For this review, take the finished solid that the model builds, in its own axes (mm). A direction names the side the tool comes from. Round coordinates to 2 decimals unless told otherwise and drop trailing zeros. Order: outer loops, then holes, each group sorted by start corner. A loop starts at its lowest first (then second) coordinate and runs counter-clockwise, first axis right, second up. Notation, with made-up numbers: M 39.25,25.5 L 46.25,25.5 A19 ccw 46.25,29.5 Z; hole C 12,72.25 d2. An arc over 180 degrees is marked long. Put each result on its own line as item: value.
Autodesk Inventor part; units mm, degrees
ref_plane "YZ Plane" through (0, 0, 0) normal (1, 0, 0) x (0, 1, 0)
ref_plane "XZ Plane" through (0, 0, 0) normal (0, 1, 0) x (-1, 0, 0)
ref_plane "XY Plane" through (0, 0, 0) normal (0, 0, 1) x (1, 0, 0)
sketch "Sketch1" plane through (0, 0, 0) normal (0, 1, 0) x (-1, 0, 0)
  line L0 (0, 0) -> (34, 0)
  line L1 (34, 0) -> (34, -2)
  line L2 (34, -2) -> (0, -2)
  line L3 (0, -2) -> (0, 0)
  line L4 (37, -5) -> (37, 3)
  line L5 (37, 3) -> (-3, 3)
  line L6 (-3, 3) -> (-3, -5)
  line L7 (-3, -5) -> (37, -5)
  dimension "d0" = 34
  dimension "d1" = 2
  dimension "d2" = 3
extrude "Extrusion1" add sketch "Sketch1" along normal blind 48 contours L0 L1 L2 L3 | L7 L6 L5 L4
sketch "Sketch3" plane through (0, 0, 0) normal (0, -1, 0) x (1, 0, 0)
  line L0 (-37, 3) -> (3, 3)
  line L1 (-37, 3) -> (3, 3)
  line L2 (3, 3) -> (3, 18)
  line L3 (3, 18) -> (-37, 18)
  line L4 (-37, 18) -> (-37, 3)
  line L5 (3, -5) -> (-37, -5)
  line L6 (-37, -5) -> (3, -5)
  line L7 (3, -5) -> (3, -20)
  line L8 (3, -20) -> (-37, -20)
  line L9 (-37, -20) -> (-37, -5)
  circle A0 centre (-27, -12.5) radius 3
  circle A1 centre (-27, 13.5) radius 3
  circle A2 centre (-7, -12.5) radius 3
  circle A3 centre (-7, 13.5) radius 3
  point P0 (0, 0)
  point P1 (3, -5)
  dimension "d5" = 40
  dimension "d6" = 15
  dimension "d7" = 40
  dimension "d8" = 15
  dimension "d9" = 6
  dimension "d10" = 10
  dimension "d11" = 7.5
  dimension "d14" = 26
  dimension "d17" = 20
extrude "Extrusion2" add sketch "Sketch3" against normal blind 6 contours L4 L3 L2 L0
sketch "Sketch5" plane through (0, 48, 0) normal (0, 1, 0) x (1, 0, 0)
  line L0 (3, 5) -> (-37, 5)
  line L1 (-37, 5) -> (3, 5)
  line L2 (3, 5) -> (3, 17)
  line L3 (3, 17) -> (-37, 17)
  line L4 (-37, 17) -> (-37, 5)
  line L5 (-32, 13) -> (-22, 13) construction
  line L6 (-32, 11.41) -> (-22, 11.41)
  line L7 (-22, 14.59) -> (-32, 14.59)
  arc A0 (-32, 14.59) -> (-32, 11.41) centre (-32, 13) ccw
  arc A1 (-22, 11.41) -> (-22, 14.59) centre (-22, 13) ccw
  line L8 (-32, 13) -> (-22, 13) construction
  line L9 (-22, 13) -> (-10.76, 13)
  line L10 (-22, 13) -> (-10.76, 13) construction
  line L11 (-10.76, 13) -> (-0.76, 13) construction
  line L12 (-10.76, 11.41) -> (-0.76, 11.41)
  line L13 (-0.76, 14.59) -> (-10.76, 14.59)
  arc A2 (-10.76, 14.59) -> (-10.76, 11.41) centre (-10.76, 13) ccw
  arc A3 (-0.76, 11.41) -> (-0.76, 14.59) centre (-0.76, 13) ccw
  point P0 (0, 0)
  point P1 (-27, 13)
  point P2 (-5.76, 13)
  point P3 (3, 5)
  dimension "d40" = 40
  dimension "d41" = 12
  dimension "d43" = 10
  dimension "d44" = 0
  dimension "d45" = 3.18
  dimension "d46" = 11.24
  dimension "d47" = 0
  dimension "d48" = 10
  dimension "d49" = 3.18
  dimension "d57" = 4
  dimension "d58" = 10
extrude "Extrusion4" add sketch "Sketch5" against normal blind 6
fillet "Fillet1" radius 3 1 edges at (-17, 42, -5)
fillet "Fillet2" radius 3 2 edges at (-17, 48, 3) (-17, 6, 3)
fillet "Fillet3" radius 3 1 edges at (-17, 6, 18)
fillet "Fillet4" radius 3 1 edges at (-17, 0, -5)
fillet "Fillet5" radius 1 2 edges at (-17, 48, -17) (-17, 42, -17)
properties part number "MagnetActuatorHolder"
(1) Add section A-A on z = -13. Give the boundary of the cut face in (x, y).
A:
outline: M -37,42 L -33.59,42 L -33.59,48 L -37,48 Z; M -20.41,42 L -12.35,42 L -12.35,48 L -20.41,48 Z; M 0.83,42 L 3,42 L 3,48 L 0.83,48 Z
(2) Add section B-B on x = -26.5. Give the boundary of the cut face in (y, z).
A:
outline: M 0,-2 A3 ccw 3,-5 L 39,-5 A3 cw 42,-8 L 42,-11.41 L 48,-11.41 L 48,0 A3 ccw 45,3 L 9,3 A3 cw 6,6 L 6,10.54 L 0,10.54 Z; M 0,16.46 L 5.62,16.46 A3 ccw 3,18 L 0,18 Z; M 42,-16 A1 ccw 43,-17 L 47,-17 A1 ccw 48,-16 L 48,-14.59 L 42,-14.59 Z
(3) Add section C-C on x = -16. Give the boundary of the cut face in (y, z), then the cut area to 3 significant figures.
A:
outline: M 0,-2 A3 ccw 3,-5 L 39,-5 A3 cw 42,-8 L 42,-16 A1 ccw 43,-17 L 47,-17 A1 ccw 48,-16 L 48,0 A3 ccw 45,3 L 9,3 A3 cw 6,6 L 6,15 A3 ccw 3,18 L 0,18 Z
area: 544 mm2
(4) For faces 1 (the face through (-6, 45, -14.59)), 2 (the face through (-17, 21, -5)), 3 (the face through (-17, 0, 8)), 4 (the face through (-17, 45, -17)), 5 (the face through (-17, 6, 11)), list the 3-axis set-ups (+Z, -Z, +X, -X, +Y, -Y) from which the entire face can be reached by the end or side of a thin tool; tool diameter is ignored.
A:
face 1: +Y, -Y
face 2: -Z, +X, -X, -Y
face 3: +Z, -Z, +X, -X, -Y
face 4: -Z, +X, -X, +Y, -Y
face 5: +Z, +X, -X, +Y
(5) Insertion check: pin 1 Ø4 at (x, z) = (-9.5, 12.5) entering from +Y; pin 2 Ø3.5 at (x, z) = (-27, 13.5) entering from -Y; pin 3 Ø18 at (x, y) = (-18, 27.5) entering from +Z; pin 4 Ø9 at (x, z) = (-26, -10) entering from -Y. Each pin has a flat end and moves straight along its axis. Give the tip position at first contact, or say it passes through.
A:
pin 1: stops at y = 6
pin 2: passes through
pin 3: stops at z = 3
pin 4: stops at y = 40.66
(6) Draft analysis for pull direction X (two halves, no side actions). For faces 6 (the face through (-37, 22, 0)), 7 (the face through (-17, 48, -8)), 8 (the face through (-12.35, 45.04, -13.03)), state which applies: released by +X, released by -X, zero draft, split by the parting line, or undercut.
A:
face 6: released by -X
face 7: zero draft
face 8: undercut
(7) To check wall thickness, follow L1, parallel to X at y = 4.5, z = 13.5; L2, parallel to Z at x = -7, y = 3.25; L3, parallel to Z at x = -2, y = 21. State the ranges of each line that lie inside material, in increasing order.
A:
L1: x = -37 to -30, -24 to -10, -4 to 3
L2: z = -5 to 10.5, 16.5 to 17.99
L3: z = -5 to 3
(8) Add section D-D on y = 14. Give the boundary of the cut face in (x, z), then the cut area to 3 significant figures.
A:
outline: M -37,-5 L 3,-5 L 3,3 L -37,3 Z
area: 320 mm2
